Autodesk Inventor part; units mm, degrees
ref_plane "YZ Plane" through (0, 0, 0) normal (1, 0, 0) x (0, 1, 0)
ref_plane "XZ Plane" through (0, 0, 0) normal (0, 1, 0) x (-1, 0, 0)
ref_plane "XY Plane" through (0, 0, 0) normal (0, 0, 1) x (1, 0, 0)
sketch "スケッチ1" plane through (0, 0, 0) normal (0, 0, 1) x (1, 0, 0)
  circle A0 centre (0, 9) radius 7.75
  line L0 (10.75, 0) -> (-58.5, 0)
  line L1 (-58.5, 0) -> (-58.5, 1.25)
  line L2 (-58.5, 1.25) -> (10.75, 1.25)
  line L3 (10.75, 1.25) -> (10.75, 0)
  circle A1 centre (0, 9) radius 10.75
  line L4 (10.75, 1.25) -> (10.75, 15.8822)
  circle A2 centre (-32, 9) radius 2.5
  circle A3 centre (-39, 9) radius 2.5
  circle A4 centre (-25, 9) radius 3.5
  circle A5 centre (-46, 9) radius 2.5
  circle A6 centre (-53, 9) radius 2.5
  circle A7 centre (-53, 9) radius 5.5
  line L5 (-58.5, 1.25) -> (-58.5, 18.7354)
  line L6 (-61.6708, 14.5) -> (12.7388, 14.5)
  point P0 (0, 0)
  point P1 (-9.2365, 14.5)
  point P2 (-58.5, 14.5)
  point P3 (10.75, 14.5)
  point P4 (9.2365, 14.5)
  dimension "d0" = 15.5
  dimension "d1" = 3
  dimension "d2" = 5
  dimension "d3" = 5
  dimension "d4" = 7
  dimension "d5" = 5
  dimension "d7" = 7
  dimension "d8" = 7
  dimension "d9" = 25
  dimension "d10" = 7
  dimension "d11" = 5
  dimension "d12" = 7
  dimension "d13" = 3
  dimension "d16" = 9
extrude "押し出し1" add sketch "スケッチ1" along normal blind 20 contours A0 L6 A1 L2 | A0 L6 A1 | L2 A1 L6 A0 | L2 A1 L0 | L6 L4 A1 | A1 L0 L1 L2 | L2 L5 A7 A5 L6 A1 | A1 L4 L2 | L2 L3 L0 A1 | A7 A5 | A7 L5 L6 picked at (-49.0972, 10.8197)
sketch "スケッチ3" plane through (0, 0, 20) normal (0, 0, 1) x (1, 0, 0)
  line L0 (-9.2365, 14.5) -> (-58.5, 14.5)
  line L1 (-58.5, 14.5) -> (-58.5, 0)
  line L2 (-58.5, 0) -> (10.75, 0)
  line L3 (10.75, 0) -> (10.75, 14.5)
  line L4 (10.75, 14.5) -> (9.2365, 14.5)
  arc A0 (9.2365, 14.5) -> (-9.2365, 14.5) centre (0, 9) ccw
  circle A1 centre (0, 9) radius 7.75
  circle A2 centre (-53, 9) radius 2.5
  circle A3 centre (-25, 9) radius 3.5
  circle A4 centre (-39, 9) radius 2.5
  circle A5 centre (-32, 9) radius 2.5
  circle A6 centre (-46, 9) radius 2.5
  line L5 (-58.5, 14.5) -> (-58.5, 0)
  line L6 (-58.5, 0) -> (-68.5, 0)
  line L7 (-68.5, 0) -> (-68.5, 14.5)
  line L8 (-68.5, 14.5) -> (-58.5, 14.5)
  line L9 (-58.5, 14.5) -> (-58.5, 0)
  line L10 (10.75, 0) -> (20.75, 0)
  line L11 (20.75, 0) -> (20.75, 14.5)
  line L12 (20.75, 14.5) -> (10.75, 14.5)
  line L13 (10.75, 14.5) -> (10.75, 0)
  point P0 (0, 0)
  dimension "d17" = 10
  dimension "d18" = 10
extrude "押し出し2" add sketch "スケッチ3" against normal up to surface (20 mm away) contours L1 L6 L7 L8 | L12 L11 L10 L3
sketch "スケッチ4" plane through (0, 0, 20) normal (0, 0, 1) x (1, 0, 0)
  line L0 (-9.2365, 14.5) -> (-68.5, 14.5)
  line L1 (-68.5, 14.5) -> (-68.5, 0)
  line L2 (-68.5, 0) -> (20.75, 0)
  line L3 (20.75, 0) -> (20.75, 14.5)
  line L4 (20.75, 14.5) -> (9.2365, 14.5)
  arc A0 (9.2365, 14.5) -> (-9.2365, 14.5) centre (0, 9) ccw
  circle A1 centre (0, 9) radius 7.75
  circle A2 centre (-53, 9) radius 2.5
  circle A3 centre (-25, 9) radius 3.5
  circle A4 centre (-39, 9) radius 2.5
  circle A5 centre (-32, 9) radius 2.5
  circle A6 centre (-46, 9) radius 2.5
  line L5 (-68.5, 0) -> (-68.5, 14.5)
  line L6 (20.75, 0) -> (20.75, 14.5)
  line L7 (-68.5, 0) -> (20.75, 0)
  line L8 (20.75, 0) -> (20.75, 9)
  line L9 (20.75, 9) -> (-68.5, 9)
  line L10 (-68.5, 9) -> (-68.5, 0)
  point P0 (0, 0)
  point P1 (-55.5, 9)
  point P2 (-68.5, 9)
  point P3 (7.75, 9)
  point P4 (-7.75, 9)
  point P5 (-28.5, 9)
  point P6 (-21.5, 9)
  point P7 (-29.5, 9)
  point P8 (-34.5, 9)
  point P9 (-36.5, 9)
  point P10 (-41.5, 9)
  point P11 (-43.5, 9)
  point P12 (-48.5, 9)
  point P13 (-50.5, 9)
extrude "押し出し3" cut sketch "スケッチ4" against normal through all contours L9 A2 A6 A4 A5 A3 A1 L3 L2 L1 | L9 A3 | A3 L9
sketch "スケッチ6" plane through (0, 0, 20) normal (0, 0, 1) x (1, 0, 0)
  line L0 (-43.5, 9) -> (-41.5, 9)
  arc A0 (-36.5, 9) -> (-41.5, 9) centre (-39, 9) ccw
  line L1 (-36.5, 9) -> (-34.5, 9)
  arc A1 (-29.5, 9) -> (-34.5, 9) centre (-32, 9) ccw
  line L2 (-29.5, 9) -> (-28.5, 9)
  arc A2 (-21.5, 9) -> (-28.5, 9) centre (-25, 9) ccw
  line L3 (-21.5, 9) -> (-7.75, 9)
  arc A3 (7.75, 9) -> (-7.75, 9) centre (0, 9) ccw
  line L4 (7.75, 9) -> (20.75, 9)
  line L5 (20.75, 9) -> (20.75, 14.5)
  line L6 (20.75, 14.5) -> (9.2365, 14.5)
  arc A4 (9.2365, 14.5) -> (-9.2365, 14.5) centre (0, 9) ccw
  line L7 (-9.2365, 14.5) -> (-68.5, 14.5)
  line L8 (-68.5, 14.5) -> (-68.5, 9)
  line L9 (-68.5, 9) -> (-55.5, 9)
  arc A5 (-50.5, 9) -> (-55.5, 9) centre (-53, 9) ccw
  line L10 (-50.5, 9) -> (-48.5, 9)
  arc A6 (-43.5, 9) -> (-48.5, 9) centre (-46, 9) ccw
  line L11 (-68.5, 14.5) -> (20.75, 14.5)
  line L12 (20.75, 14.5) -> (20.75, 16.5)
  line L13 (20.75, 16.5) -> (-68.5, 16.5)
  line L14 (-68.5, 16.5) -> (-68.5, 14.5)
  point P0 (0, 0)
  point P1 (7.7015, 16.5)
  point P2 (-7.7015, 16.5)
  dimension "d33" = 2
extrude "押し出し4" add sketch "スケッチ6" against normal up to surface (20 mm away) contours L14 L13 A4 L7 | L13 L12 L6 A4
sketch "スケッチ7" plane through (7.7015, 16.5, 20) normal (0, 1, 0) x (1, 0, 0)
  line L0 (0, 20) -> (13.0485, 20)
  line L1 (0, 0) -> (0, 20)
  line L2 (13.0485, 0) -> (0, 0)
  line L3 (13.0485, 0) -> (13.0485, 20)
  line L4 (-76.2015, 20) -> (-15.4029, 20)
  line L5 (-76.2015, 0) -> (-76.2015, 20)
  line L6 (-15.4029, 0) -> (-76.2015, 0)
  line L7 (-15.4029, 20) -> (-15.4029, 0)
  point P0 (-7.7015, 20)
  point P1 (8.0485, 10)
  point P2 (-23.4515, 10)
  point P3 (-71.2015, 10)
  dimension "d36" = 5
  dimension "d37" = 10
  dimension "d38" = 10
  dimension "d39" = 15.75
  dimension "d40" = 5
hole "穴2" at (15.75, 16.5, 10) at (-15.75, 16.5, 10) at (-63.5, 16.5, 10) direction (0, -1, 0) diameter 4.3 end through all
chamfer "面取り1" distance 2 angle 45 2 edges at (20.75, 16.5, 10) (-68.5, 16.5, 10)
chamfer "面取り2" distance 2 angle 45 4 edges at (20.75, 11.75, 0) (20.75, 11.75, 20) (-68.5, 11.75, 0) (-68.5, 11.75, 20)
properties part number "C_Unit_Cable_Holder_A"
Design review of the part built by this model. Coordinates are the model's own, in mm. A direction names the side the tool comes from. Coordinates: 2 decimals unless noted, no trailing zeros. Order: outer loops, then holes, each group sorted by start corner. A loop starts at its lowest first (then second) coordinate and runs counter-clockwise, first axis right, second up. Notation, with made-up numbers: (-18.5, -11) -> (-9.5, -11) arc R15 ccw to (-9.5, 15) -> close; hole circle Ø5 at (16.5, -24.75). An arc over 180 degrees is marked (long way). One line per item, written item: value. Start each with the question number.
Q1. Tool access review of faces 4 (the flat face through (-37, 16.5, 10)), 5 (the flat face through (13, 16.5, 10)), 6 (the flat face through (19.74, 11.86, 19.01)): name each direction out of +Z, -Z, +X, -X, +Y, -Y from which nothing blocks a thin tool from reaching the whole face with its end or side.
Q2. For probe 1 along Z at (x, y) = (-15.75, 11); probe 2 along X at (y, z) = (13.25, 10); probe 3 along X at (y, z) = (13, 10), list the stretches that pass through material, from the lowest coordinate up.
Q3. Take a section at D-D, the plane x = -46. State the section outline as (y, z) points.
Q4. Take a section at A-A, the plane z = 10. Give the number of separate pieces and of enclosed holes in the cut face, then the cut area to 3 significant figures.
Q5. Mouldability with a two-part tool opening along Z and no side actions: class faces 1 (the flat face through (20.75, 12, 10)), 2 (the flat face through (-24, 13, 20)), 3 (the cylindrical face through (17.85, 12.7, 9.53)) as pulls with the +Z half, pulls with the -Z half, needs draft (parallel to the pull), parting line crosses it, or undercut.
Q6. Take a section at B-B, the plane x = -25. State the section outline as (y, z) points.
Q7. Insertion check: pin 1 Ø5.5 at (x, z) = (-63.5, 10) entering from +Y. The pin has a flat end and moves straight along its axis. Give the tip position at first contact, or say it passes through.
Q8. Take a section at C-C, the plane z = 14.75. State the section outline as (x, y) points, then the cut area to 3 significant figures.
Values follow:
1. face 4: +Z, -Z, -X, +Y
1. face 5: +Z, -Z, +X, +Y
1. face 6: +Z, +X, +Y, -Y
2. probe 1: z = 0 to 7.85, 12.15 to 20
2. probe 2: x = -68.5 to -65.65, -61.35 to -17.9, -13.6 to -6.48, 6.48 to 13.6, 17.9 to 20.75
2. probe 3: x = -68.5 to -65.65, -61.35 to -17.9, -13.6 to -6.64, 6.64 to 13.6, 17.9 to 20.75
3. outline: (11.5, 0) -> (16.5, 0) -> (16.5, 20) -> (11.5, 20) -> close
4. separate pieces: 4
4. enclosed holes: 0
4. area: 450 mm2
5. face 1: needs draft
5. face 2: pulls with the +Z half
5. face 3: undercut
6. outline: (12.5, 0) -> (16.5, 0) -> (16.5, 20) -> (12.5, 20) -> close
7. pin 1: stops at y = 16.5
8. outline: (-68.5, 9) -> (-55.5, 9) arc R2.5 cw to (-50.5, 9) -> (-48.5, 9) arc R2.5 cw to (-43.5, 9) -> (-41.5, 9) arc R2.5 cw to (-36.5, 9) -> (-34.5, 9) arc R2.5 cw to (-29.5, 9) -> (-28.5, 9) arc R3.5 cw to (-21.5, 9) -> (-7.75, 9) arc R7.75 cw to (7.75, 9) -> (20.75, 9) -> (20.75, 14.5) -> (18.75, 16.5) -> (7.7, 16.5) arc R10.75 ccw to (-7.7, 16.5) -> (-66.5, 16.5) -> (-68.5, 14.5) -> close
8. area: 547 mm2
